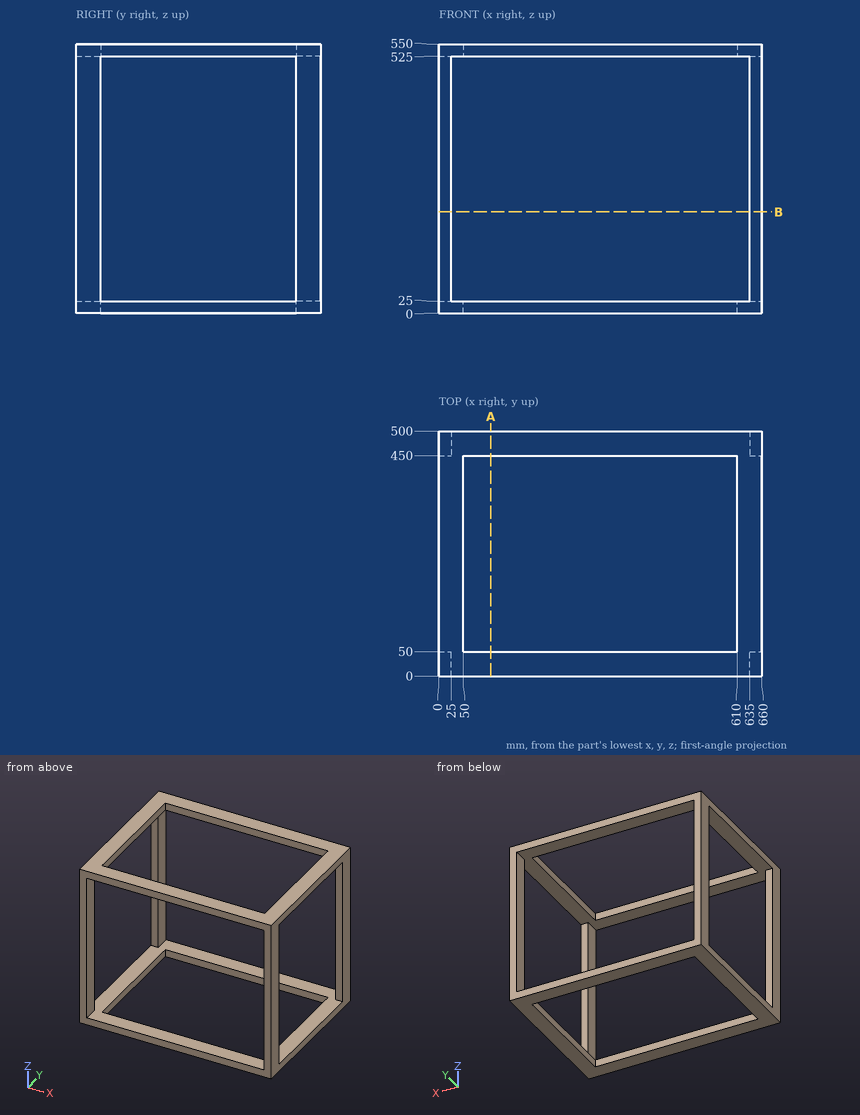
Part print with two shaded views. Sizes in mm from the minimum x, y, z corner. Coordinates: 2 decimals unless noted, no trailing zeros. Order: outer loops, then holes, each group sorted by start corner. A loop starts at its lowest first (then second) coordinate and runs counter-clockwise, first axis right, second up. Notation, with made-up numbers: (32.25, 62) - (61.25, 62) arc R13 ccw to (61.25, 85) - close; hole circle Ø7 at (57, -16). An arc over 180 degrees is marked (long way). Write item = value, one per line. Start each with the question number.
1) Wall check: line 1 along Z through (x, y) = (183, 27); line 2 along Y through (x, z) = (299, 526.5); line 3 along X through (y, z) = (476.5, 213). Give the ranges that are in metal, low to high. Write a range as from..to.
2) Saw through at B-B on z = 207. Write the cut outline in (x, y), then the cut area to 3 significant figures.
3) Saw through at A-A on x = 106.5. Write the cut outline in (y, z).
From the geometry:
q1.line_1 = 0..25, 525..550
q1.line_2 = 0..50, 450..500
q1.line_3 = 0..25, 635..660
q2.outline = (0, 0) - (25, 0) - (25, 50) - (0, 50) - close; (0, 450) - (25, 450) - (25, 500) - (0, 500) - close; (635, 0) - (660, 0) - (660, 50) - (635, 50) - close; (635, 450) - (660, 450) - (660, 500) - (635, 500) - close
q2.area = 5,000 mm^2
q3.outline = (0, 0) - (50, 0) - (50, 25) - (0, 25) - close; (0, 525) - (50, 525) - (50, 550) - (0, 550) - close; (450, 0) - (500, 0) - (500, 25) - (450, 25) - close; (450, 525) - (500, 525) - (500, 550) - (450, 550) - close
